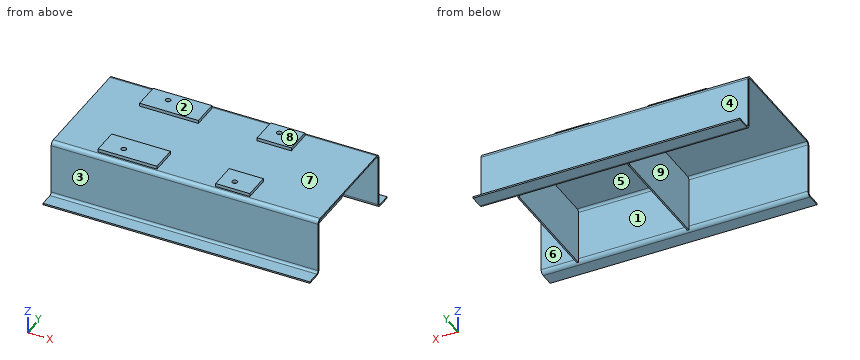
```python
from build123d import *

# Parameters (mm, degrees)
F1_DEPTH = 1066.8
F2_W     = 12.7
F2_H     = 914.4
F3_DEPTH = 450.85
F4_W     = 469.9
F4_H     = 209.55
F4_R     = 20.6375
F4_W_2   = 273.05
F5_DEPTH = 25.4


with BuildPart() as f1:
    # F0 (on Right) → F1 (new body, symmetric)
    with BuildSketch(Plane.YZ):
        with BuildLine():
            ThreePointArc((457.2, 31.75), (466.49936, 9.29936), (488.95, 0))
            Line((488.95, 0), (596.9, 0))
            Line((596.9, 0), (596.9, 12.7))
            Line((596.9, 12.7), (488.95, 12.7))
            ThreePointArc((488.95, 12.7), (475.479616, 18.279616), (469.9, 31.75))
            Line((469.9, 31.75), (469.9, 431.8))
            ThreePointArc((469.9, 431.8), (460.60064, 454.25064), (438.15, 463.55))
            Line((438.15, 463.55), (0, 463.55))
            Line((0, 463.55), (-438.15, 463.55))
            ThreePointArc((-438.15, 463.55), (-460.60064, 454.25064), (-469.9, 431.8))
            Line((-469.9, 431.8), (-469.9, 31.75))
            ThreePointArc((-469.9, 31.75), (-475.479616, 18.279616), (-488.95, 12.7))
            Line((-488.95, 12.7), (-596.9, 12.7))
            Line((-596.9, 12.7), (-596.9, 0))
            Line((-596.9, 0), (-488.95, 0))
            ThreePointArc((-488.95, 0), (-466.49936, 9.29936), (-457.2, 31.75))
            Line((-457.2, 31.75), (-457.2, 431.8))
            ThreePointArc((-457.2, 431.8), (-451.620384, 445.270384), (-438.15, 450.85))
            Line((-438.15, 450.85), (0, 450.85))
            Line((0, 450.85), (438.15, 450.85))
            ThreePointArc((438.15, 450.85), (451.620384, 445.270384), (457.2, 431.8))
            Line((457.2, 431.8), (457.2, 31.75))
        make_face()
    extrude(amount=F1_DEPTH, both=True)

    # F2 (on face) → F3 (join, through all)
    with BuildSketch(Plane(origin=(0, 0, 450.85), x_dir=(1, 0, 0), z_dir=(0, 0, -1))):
        with Locations((-107.95, 0)):
            Rectangle(F2_W, F2_H)
        with Locations((774.7, 0)):
            Rectangle(F2_W, F2_H)
    extrude(amount=F3_DEPTH)

    # F4 (on face) → F5 (join)
    with BuildSketch(Plane.XY.offset(463.55)):
        with Locations((-479.552, 320.675)):
            Rectangle(F4_W, F4_H)
        with Locations((-552.45, 342.9)):
            Circle(F4_R, mode=Mode.SUBTRACT)
        with Locations((361.823, 320.675)):
            Rectangle(F4_W_2, F4_H)
        with Locations((336.55, 342.9)):
            Circle(F4_R, mode=Mode.SUBTRACT)
        with Locations((361.823, -320.675)):
            Rectangle(F4_W_2, F4_H)
        with Locations((336.55, -342.9)):
            Circle(F4_R, mode=Mode.SUBTRACT)
        with Locations((-479.552, -320.675)):
            Rectangle(F4_W, F4_H)
        with Locations((-552.45, -342.9)):
            Circle(F4_R, mode=Mode.SUBTRACT)
    extrude(amount=F5_DEPTH)


solid = f1.part
```
Could you check a few things on this model? Use its own coordinates, in mm. Face numbers are marked on the shaded views. A direction names the side the tool comes from. Coordinates: 2 decimals unless noted, no trailing zeros. Write each loop counter-clockwise with the first axis right and the second up, starting at its lowest first coordinate (ties: lowest second). Pieces come first, ordered by that corner, then holes. Notation, with made-up numbers: (65, 18.25) -> (123, 18.25) arc R14 cw to (123, 45.25) -> close; hole circle Ø1 at (-22, -5). An arc over 180 degrees is marked (long way). Return JSON: item names as keys, results as strings.
(1) I need wall thicknesses on L1, parallel to Y at x = -552.45, z = 470; L2, parallel to X at y = 72, z = 361. Which ranges of each line are inside material? Lowest first, please.
Numbers:
{"L1": "y = -425.45 to -363.54, -322.26 to -215.9, 215.9 to 322.26, 363.54 to 425.45", "L2": "x = -114.3 to -101.6, 768.35 to 781.05"}
(2) Imagine slicing it at B-B, the plane y = 299.5. Please give me the cut outline in (x, z), then the cut area to 3 significant figures.
Numbers:
{"outline": "(-1066.8, 450.85) -> (-114.3, 450.85) -> (-114.3, 0) -> (-101.6, 0) -> (-101.6, 450.85) -> (768.35, 450.85) -> (768.35, 0) -> (781.05, 0) -> (781.05, 450.85) -> (1066.8, 450.85) -> (1066.8, 463.55) -> (498.35, 463.55) -> (498.35, 488.95) -> (225.3, 488.95) -> (225.3, 463.55) -> (-244.6, 463.55) -> (-244.6, 488.95) -> (-714.5, 488.95) -> (-714.5, 463.55) -> (-1066.8, 463.55) -> close", "area": "57,400 mm2"}
(3) Which directions (+Z, -Z, +X, -X, +Y, -Y) give clear straight access to the entire face, cutting with the end or side of a thin tool? Please do the marked faces 5, 6, 7, 8 and 9.
Numbers:
{"face 5": "-Z", "face 6": "-Z, +X", "face 7": "+Z", "face 8": "+Z, +X, -X, +Y, -Y", "face 9": "-Z, -X"}
(4) Imagine slicing it at D-D, the plane y = -342.9. Please give me the cut outline in (x, z), then the cut area to 3 significant figures.
Numbers:
{"outline": "(-1066.8, 450.85) -> (-114.3, 450.85) -> (-114.3, 0) -> (-101.6, 0) -> (-101.6, 450.85) -> (768.35, 450.85) -> (768.35, 0) -> (781.05, 0) -> (781.05, 450.85) -> (1066.8, 450.85) -> (1066.8, 463.55) -> (498.35, 463.55) -> (498.35, 488.95) -> (357.19, 488.95) -> (357.19, 463.55) -> (315.91, 463.55) -> (315.91, 488.95) -> (225.3, 488.95) -> (225.3, 463.55) -> (-244.6, 463.55) -> (-244.6, 488.95) -> (-531.81, 488.95) -> (-531.81, 463.55) -> (-573.09, 463.55) -> (-573.09, 488.95) -> (-714.5, 488.95) -> (-714.5, 463.55) -> (-1066.8, 463.55) -> close", "area": "55,300 mm2"}
(5) Imagine slicing it at A-A, the plane z = 301.5. Please give me the cut outline in (x, y).
Numbers:
{"outline": "(-1066.8, -469.9) -> (1066.8, -469.9) -> (1066.8, -457.2) -> (781.05, -457.2) -> (781.05, 457.2) -> (1066.8, 457.2) -> (1066.8, 469.9) -> (-1066.8, 469.9) -> (-1066.8, 457.2) -> (-114.3, 457.2) -> (-114.3, -457.2) -> (-1066.8, -457.2) -> close; hole (-101.6, -457.2) -> (768.35, -457.2) -> (768.35, 457.2) -> (-101.6, 457.2) -> close"}
(6) Imagine slicing it at C-C, the plane x = -292. Please give me the cut outline in (y, z), then the cut area to 3 significant figures.
Numbers:
{"outline": "(-596.9, 0) -> (-488.95, 0) arc R31.75 ccw to (-457.2, 31.75) -> (-457.2, 431.8) arc R19.05 cw to (-438.15, 450.85) -> (438.15, 450.85) arc R19.05 cw to (457.2, 431.8) -> (457.2, 31.75) arc R31.75 ccw to (488.95, 0) -> (596.9, 0) -> (596.9, 12.7) -> (488.95, 12.7) arc R19.05 cw to (469.9, 31.75) -> (469.9, 431.8) arc R31.75 ccw to (438.15, 463.55) -> (425.45, 463.55) -> (425.45, 488.95) -> (215.9, 488.95) -> (215.9, 463.55) -> (-215.9, 463.55) -> (-215.9, 488.95) -> (-425.45, 488.95) -> (-425.45, 463.55) -> (-438.15, 463.55) arc R31.75 ccw to (-469.9, 431.8) -> (-469.9, 31.75) arc R19.05 cw to (-488.95, 12.7) -> (-596.9, 12.7) -> close", "area": "36,700 mm2"}
(7) We'd pull the mould along Y, two halves only. Please class the marked faces 1, 2, 3 and 4: +Y half, -Y half, draft (parallel to the pull), parting line (faces both ways), or undercut.
Numbers:
{"face 1": "undercut", "face 2": "draft", "face 3": "-Y half", "face 4": "+Y half"}
(8) I'm going to push flat-ended pins straight in: pin 1 (7.5 mm diameter, centred on x = -473.5, z = 478, fed in from +Y); pin 2 (10 mm diameter, centred on x = -229.5, z = 367, fed in from -Y); pin 3 (4 mm diameter, centred on x = 327, z = 332, fed in from +Y). Where does each tip first touch, or does it pass through?
Numbers:
{"pin 1": "stops at y = 425.45", "pin 2": "stops at y = -469.9", "pin 3": "stops at y = 469.9"}
